from build123d import *

# Parameters (mm, degrees)
F1_DEPTH = 3
F2_R     = 3.5
F2_W     = 1.3
F2_H     = 2.8
F3_DEPTH = 3.001
F4_R     = 1.05
F4_R_2   = 1.6
F5_DEPTH = 3.001


with BuildPart() as f1:
    # F0 (on Top) → F1 (new body)
    with BuildSketch(Plane.XY):
        with BuildLine():
            Line((35, 65), (-35, 65))
            ThreePointArc((-35, 65), (-38.535534, 63.535534), (-40, 60))
            Line((-40, 60), (-40, -60))
            ThreePointArc((-40, -60), (-38.535534, -63.535534), (-35, -65))
            Line((-35, -65), (35, -65))
            ThreePointArc((35, -65), (38.535534, -63.535534), (40, -60))
            Line((40, -60), (40, 60))
            ThreePointArc((40, 60), (38.535534, 63.535534), (35, 65))
        make_face()
    extrude(amount=F1_DEPTH)

    # F2 (on face) → F3 (cut, through all)
    with BuildSketch(Plane.XY.offset(3)):
        with Locations((0, 15)):
            Circle(F2_R)
        with Locations((0, -35)):
            Circle(F2_R)
        with Locations((-8, 15)):
            Rectangle(F2_W, F2_H)
        Polygon((-2.462564, 22.065287), (-3.112564, 23.19112), (-5.537436, 21.79112), (-4.887436, 20.665287), align=None)
        Polygon((4.887436, 20.665287), (5.537436, 21.79112), (3.112564, 23.19112), (2.462564, 22.065287), align=None)
        with Locations((8, 15)):
            Rectangle(F2_W, F2_H)
        Polygon((2.462564, 7.934713), (3.112564, 6.80888), (5.537436, 8.20888), (4.887436, 9.334713), align=None)
        Polygon((-4.887436, 9.334713), (-5.537436, 8.20888), (-3.112564, 6.80888), (-2.462564, 7.934713), align=None)
        with Locations((-8, -35)):
            Rectangle(F2_W, F2_H)
        Polygon((-4.887436, -40.665287), (-5.537436, -41.79112), (-3.112564, -43.19112), (-2.462564, -42.065287), align=None)
        Polygon((2.462564, -42.065287), (3.112564, -43.19112), (5.537436, -41.79112), (4.887436, -40.665287), align=None)
        with Locations((8, -35)):
            Rectangle(F2_W, F2_H)
        Polygon((4.887436, -29.334713), (5.537436, -28.20888), (3.112564, -26.80888), (2.462564, -27.934713), align=None)
        Polygon((-2.462564, -27.934713), (-3.112564, -26.80888), (-5.537436, -28.20888), (-4.887436, -29.334713), align=None)
    extrude(amount=-F3_DEPTH, mode=Mode.SUBTRACT)

    # F4 (on face) → F5 (cut, through all)
    with BuildSketch(Plane.XY.offset(3)):
        with Locations((-28.5, 0.25)):
            Circle(F4_R)
        with Locations((28.5, 0.25)):
            Circle(F4_R)
        with Locations((28.5, -20.25)):
            Circle(F4_R)
        with Locations((-28.5, -20.25)):
            Circle(F4_R)
        with Locations((-35, 60)):
            Circle(F4_R_2)
        with Locations((35, 60)):
            Circle(F4_R_2)
        with Locations((35, -60)):
            Circle(F4_R_2)
        with Locations((-35, -60)):
            Circle(F4_R_2)
    extrude(amount=-F5_DEPTH, mode=Mode.SUBTRACT)


solid = f1.part
Design review of the part built by this model. Coordinates are the model's own, in mm. A direction names the side the tool comes from. Round coordinates to 2 decimals unless told otherwise and drop trailing zeros. Write each loop counter-clockwise with the first axis right and the second up, starting at its lowest first coordinate (ties: lowest second). Pieces come first, ordered by that corner, then holes. Notation, with made-up numbers: (-19, 2) - (29, 2) arc R14 cw to (29, 16) - close; hole circle Ø8 at (22.25, 61). An arc over 180 degrees is marked (long way). Return JSON: item names as keys, results as strings. Group by question number.
Item 1: We need section A-A on y = 15. Write out the cut boundary in (x, z).
Item 2: For probe 1 along Y at (x, z) = (-7.5, 2.45); probe 2 along Y at (x, z) = (35, 1.2); probe 3 along X at (y, z) = (-20, 0.2), list the stretches that pass through material, from the lowest coordinate up. Write a range as [from, to].
Item 3: Machinability: for faces 4 (the face through (-1, 1, 0)), 5 (the face through (8.65, -35, 2)), which of the approach directions +Z, -Z, +X, -X, +Y, -Y give a long, thin tool a straight path to every point of the face, cutting with its end or side? Answer none if there is none.
Item 4: We need section B-B on z = 0.55. Give the number of separate pieces and of enclosed holes in the cut face, and give its area (3 significant figures).
Item 5: The part is to be moulded in two halves that separate along X. For faces 1 (the face through (-38, 64, 1)), 2 (the face through (38, -64, 1)), 3 (the face through (8.65, 15, 2)), say which applies: pulls with the +X half, pulls with the -X half, needs draft (parallel to the pull), parting line crosses it, or undercut.
Model answer:
{
 "1": {"outline": "(-40, 0) - (-8.65, 0) - (-8.65, 3) - (-40, 3) - close; (-7.35, 0) - (-3.5, 0) - (-3.5, 3) - (-7.35, 3) - close; (3.5, 0) - (7.35, 0) - (7.35, 3) - (3.5, 3) - close; (8.65, 0) - (40, 0) - (40, 3) - (8.65, 3) - close"},
 "2": {"probe 1": "y = [-65, -36.4], [-33.6, 13.6], [16.4, 65]", "probe 2": "y = [-65, -61.6], [-58.4, 58.4], [61.6, 65]", "probe 3": "x = [-40, -29.52], [-27.48, 27.48], [29.52, 40]"},
 "3": {"face 4": "-Z, +X, -X, +Y, -Y", "face 5": "+Z, -Z"},
 "4": {"separate pieces": "1", "enclosed holes": "22", "area": "10,200 mm²"},
 "5": {"face 1": "pulls with the -X half", "face 2": "pulls with the +X half", "face 3": "undercut"}
}
